Input: dimensioned drawing with shaded views. Units: mm. Origin: part minimum x, y, z. A direction names the side the tool comes from. Round coordinates to 2 decimals unless told otherwise and drop trailing zeros. Order: outer loops, then holes, each group sorted by start corner. A loop starts at its lowest first (then second) coordinate and runs counter-clockwise, first axis right, second up. Notation, with made-up numbers: (85, -30.5) - (98, -30.5) arc R24 cw to (98, -0.5) - close; hole circle Ø3 at (26.5, -6). An arc over 180 degrees is marked (long way). One line per item, written item: value. Start each with the question number.
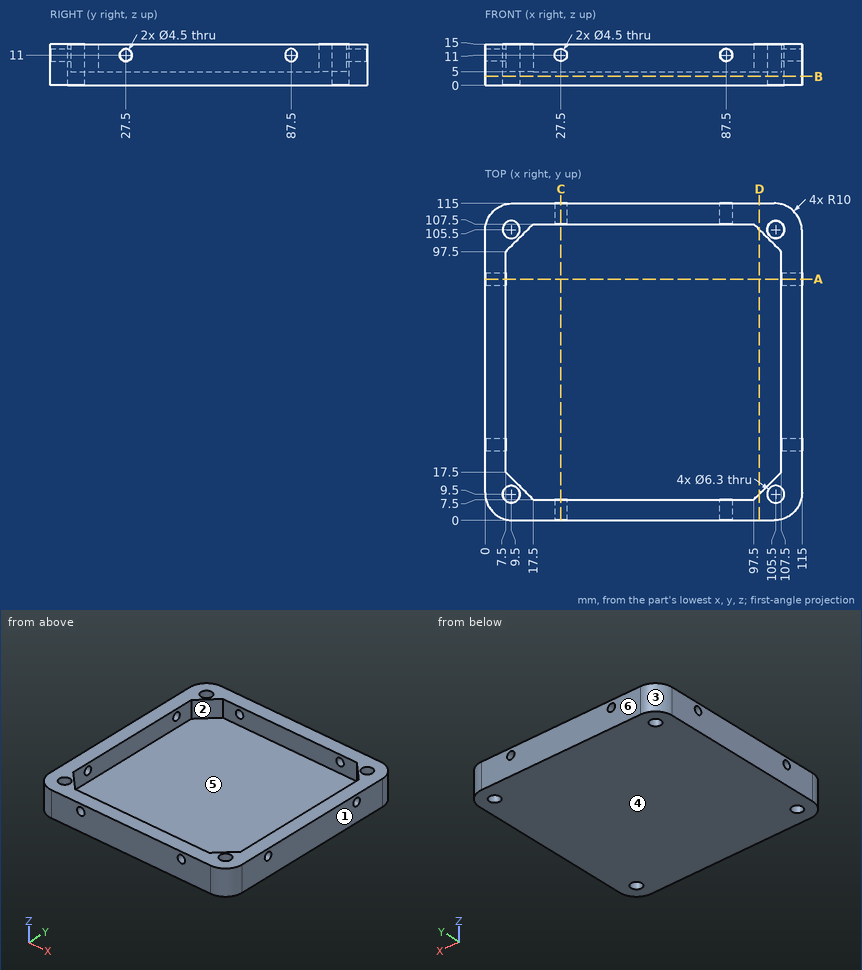
1. Section D-D (x = 99.5). Return the cut outline in (y, z).
2. Line query: line 1 (Z direction, x = 87.5, y = 112); line 2 (X direction, y = 36, z = 11.75). Output: solid intervals per line, ascending. Write a range as from..to.
3. Section B-B (z = 3.25). Return the cut outline in (x, y), then the cut area to 3 significant figures.
4. Section A-A (y = 87.5). Return the cut outline in (x, z), then the cut area to 4 significant figures.
5. Pull-direction query (X, two-part tool) for the marked faces 1, 2, 3 and 4; classes: released by +X, released by -X, zero draft, split by the parting line, or undercut.
6. Pin query (flat end, axial travel): pin 1 (1.5 mm diameter, centred on x = 68.5, y = 33, fed in from +Z); pin 2 (3 mm diameter, centred on y = 82.5, z = 13.5, fed in from -X). Return the tip coordinate at first contact, or that it passes through.
7. Set-up query: the marked faces 5 and 6. Return all of +Z, -Z, +X, -X, +Y, -Y with unobstructed straight access to the full face (end or side cutting, diameter ignored); none if empty.
Solved:
1. outline: (0, 0) - (115, 0) - (115, 15) - (105.5, 15) - (105.5, 5) - (9.5, 5) - (9.5, 15) - (0, 15) - close
2. line 1: z = 0..8.75, 13.25..15
2. line 2: x = 0..7.5, 107.5..115
3. outline: (0, 10) arc R10 ccw to (10, 0) - (105, 0) arc R10 ccw to (115, 10) - (115, 105) arc R10 ccw to (105, 115) - (10, 115) arc R10 ccw to (0, 105) - close; hole circle Ø6.3 at (9.5, 9.5); hole circle Ø6.3 at (9.5, 105.5); hole circle Ø6.3 at (105.5, 9.5); hole circle Ø6.3 at (105.5, 105.5)
3. area: 13,000 mm²
4. outline: (0, 0) - (115, 0) - (115, 8.75) - (107.5, 8.75) - (107.5, 5) - (7.5, 5) - (7.5, 8.75) - (0, 8.75) - close; (0, 13.25) - (7.5, 13.25) - (7.5, 15) - (0, 15) - close; (107.5, 13.25) - (115, 13.25) - (115, 15) - (107.5, 15) - close
4. area: 657.5 mm²
5. face 1: released by +X
5. face 2: undercut
5. face 3: released by -X
5. face 4: zero draft
6. pin 1: stops at z = 5
6. pin 2: stops at x = 0
7. face 5: +Z
7. face 6: +Z, -Z, +X, -X, +Y
